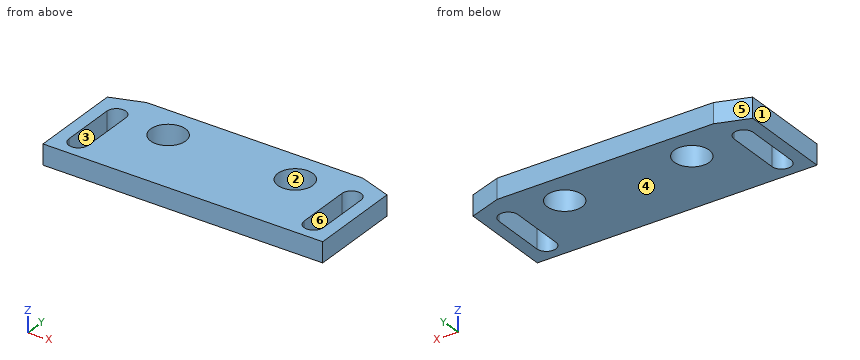
from build123d import *

# Parameters (mm, degrees)
SKETCH1_R           = 2.75
BOSS_EXTRUDE1_DEPTH = 3.18


with BuildPart() as part:
    # Sketch1 → Boss-Extrude1 (new body)
    with BuildSketch(Plane.XY):
        Polygon((-22, -26.101619014), (22, -26.101619014), (22, -11.5), (17, -9.761557864), (-17, -9.761557864), (-22, -11.5), align=None)
        with Locations(Location((10, -15, 0), (0, 0, 180))):
            Circle(SKETCH1_R, mode=Mode.SUBTRACT)
        with Locations(Location((-10, -15, 0), (0, 0, 180))):
            Circle(SKETCH1_R, mode=Mode.SUBTRACT)
        with BuildLine():
            Line((20, -23.101619014), (20, -14.498380986))
            ThreePointArc((20, -14.498380986), (18.5, -12.998380986), (17, -14.498380986))
            Line((17, -14.498380986), (17, -23.101619014))
            ThreePointArc((17, -23.101619014), (18.5, -24.601619014), (20, -23.101619014))
        make_face(mode=Mode.SUBTRACT)
        with BuildLine():
            Line((-20, -23.101619014), (-20, -14.498380986))
            ThreePointArc((-20, -14.498380986), (-18.5, -12.998380986), (-17, -14.498380986))
            Line((-17, -14.498380986), (-17, -23.101619014))
            ThreePointArc((-17, -23.101619014), (-18.5, -24.601619014), (-20, -23.101619014))
        make_face(mode=Mode.SUBTRACT)
    extrude(amount=BOSS_EXTRUDE1_DEPTH)


solid = part.part
CAD build for the part. Positions are in the model's coordinates, mm. Face numbers are marked on the shaded views. A direction names the side the tool comes from. Round coordinates to 2 decimals unless told otherwise and drop trailing zeros. Order: outer loops, then holes, each group sorted by start corner. A loop starts at its lowest first (then second) coordinate and runs counter-clockwise, first axis right, second up. Notation, with made-up numbers: (58.5, 27) - (92.5, 27) arc R23 ccw to (92.5, 54) - close; hole circle Ø7 at (5, -8). An arc over 180 degrees is marked (long way). Return JSON: item names as keys, results as strings.
(1) Tool access for the marked faces 5 and 6: list every direction of +Z, -Z, +X, -X, +Y, -Y with a clear straight run to the whole face (end or side of a thin tool).
Answer key:
{"face 5": "+Z, -Z, -X, +Y", "face 6": "+Z, -Z"}
(2) Cut at C-C (x = -10). Give the cut face in (y, z), then the cut area to 3 significant figures.
Answer key:
{"outline": "(-26.1, 0) - (-17.75, 0) - (-17.75, 3.18) - (-26.1, 3.18) - close; (-12.25, 0) - (-9.76, 0) - (-9.76, 3.18) - (-12.25, 3.18) - close", "area": "34.5 mm^2"}
(3) Pull direction X, two halves, no side cores. Call the marked faces 1, 2, 3 and 4: +X half, -X half, draft (parallel to the pull), parting line (faces both ways), or undercut.
Answer key:
{"face 1": "-X half", "face 2": "undercut", "face 3": "undercut", "face 4": "draft"}
(4) Cut at D-D (y = -18.5). Give the cut face in (x, z).
Answer key:
{"outline": "(-22, 0) - (-20, 0) - (-20, 3.18) - (-22, 3.18) - close; (-17, 0) - (17, 0) - (17, 3.18) - (-17, 3.18) - close; (20, 0) - (22, 0) - (22, 3.18) - (20, 3.18) - close"}
(5) Cut at A-A (y = -15). Give the cut face in (x, z).
Answer key:
{"outline": "(-22, 0) - (-20, 0) - (-20, 3.18) - (-22, 3.18) - close; (-17, 0) - (-12.75, 0) - (-12.75, 3.18) - (-17, 3.18) - close; (-7.25, 0) - (7.25, 0) - (7.25, 3.18) - (-7.25, 3.18) - close; (12.75, 0) - (17, 0) - (17, 3.18) - (12.75, 3.18) - close; (20, 0) - (22, 0) - (22, 3.18) - (20, 3.18) - close"}
(6) Cut at B-B (z = 1.6). Give the cut face in (x, y).
Answer key:
{"outline": "(-22, -26.1) - (22, -26.1) - (22, -11.5) - (17, -9.76) - (-17, -9.76) - (-22, -11.5) - close; hole (-20, -23.1) arc R1.5 ccw to (-17, -23.1) - (-17, -14.5) arc R1.5 ccw to (-20, -14.5) - close; hole circle Ø5.5 at (-10, -15); hole circle Ø5.5 at (10, -15); hole (17, -23.1) arc R1.5 ccw to (20, -23.1) - (20, -14.5) arc R1.5 ccw to (17, -14.5) - close"}
(7) Wall check: probe 1 along X at (y, z) = (-15, 1.95); probe 2 along X at (y, z) = (-21.75, 1.95); probe 3 along Y at (x, z) = (10, 1.4). Give the ranges that are in metal, low to high. Write a range as from..to.
Answer key:
{"probe 1": "x = -22..-20, -17..-12.75, -7.25..7.25, 12.75..17, 20..22", "probe 2": "x = -22..-20, -17..17, 20..22", "probe 3": "y = -26.1..-17.75, -12.25..-9.76"}
